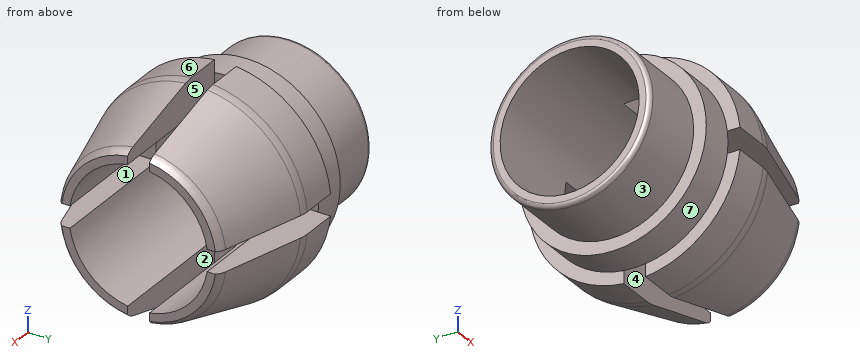
from build123d import *

# Parameters (mm, degrees)
F2_W          = 2.032
F2_H          = 3.556
F2_W_2        = 3.556
F2_H_2        = 2.032
F3_DEPTH      = 25.4
F3_DEPTH_BACK = 4.3434


# Not quite as in the source:
# - a feature names something its author has since deleted; it is built from what else it names


with BuildPart() as f1:
    # F0 (on Front) → F1 (revolve)
    with BuildSketch(Plane.XZ):
        with BuildLine():
            ThreePointArc((8.3732076521, 7.2620277332), (8.0243377529, 7.5505761386), (7.608205325, 7.728913435))
            Line((7.608205325, 7.728913435), (-0.1130385595, 9.7978144985))
            ThreePointArc((-0.1130385595, 9.7978144985), (-0.5203683675, 9.8788374349), (-0.9347890277, 9.906))
            Line((-0.9347890277, 9.906), (-4.3267923479, 9.906))
            Line((-4.3267923479, 9.906), (-4.3267923479, 8.73125))
            Line((-4.3267923479, 8.73125), (-7.5017923479, 8.73125))
            Line((-7.5017923479, 8.73125), (-7.5017923479, 7.5438))
            Line((-7.5017923479, 7.5438), (-13.4549173479, 7.5438))
            ThreePointArc((-13.4549173479, 7.5438), (-13.7355503517, 7.4275580038), (-13.8517923479, 7.146925))
            Line((-13.8517923479, 7.146925), (-13.8517923479, 6.5024))
            Line((-13.8517923479, 6.5024), (8.3732076521, 6.5024))
            Line((8.3732076521, 6.5024), (8.3732076521, 7.2620277332))
        make_face()
    revolve(axis=Axis((-0.2325048039, 0, 0), (1, 0, 0)))

    # F2 (on Right) → F3 (cut, two sides)
    with BuildSketch(Plane.YZ) as f3_sk:
        with Locations((0, -8.1534)):
            Rectangle(F2_W, F2_H)
        with Locations((0, 8.1534)):
            Rectangle(F2_W, F2_H)
        with Locations((-8.1534, 0)):
            Rectangle(F2_W_2, F2_H_2)
        with Locations((8.1534, 0)):
            Rectangle(F2_W_2, F2_H_2)
    extrude(amount=F3_DEPTH, mode=Mode.SUBTRACT)
    extrude(f3_sk.sketch, amount=-F3_DEPTH_BACK, mode=Mode.SUBTRACT)


solid = f1.part
The listing builds one solid part. Answer for the finished solid, in the listing's coordinates (mm). Face numbers are marked on the shaded views. A direction names the side the tool comes from. Round coordinates to 2 decimals unless told otherwise and drop trailing zeros. Write each loop counter-clockwise with the first axis right and the second up, starting at its lowest first coordinate (ties: lowest second). Pieces come first, ordered by that corner, then holes. Notation, with made-up numbers: M 76.5,38.25 L 125.5,38.25 A15 cw 125.5,53.25 Z; hole C 81.5,14.5 d6. An arc over 180 degrees is marked long. Write each question's results on one line, items separated by ' | '. Start each with the question number.
Item 1: The mould has two halves that part along Y. Classify the marked faces 4, 5, 6 and 7: +Y half, -Y half, draft (parallel to the pull), parting line (faces both ways), or undercut.
Item 2: Find section D-D on x = -7. Write down the section's boundary in (y, z), and give its area (3 significant figures).
Item 3: Find section A-A on z = 0. Write down the section's boundary in (x, y).
Item 4: Find section B-B on x = 7. Write down the section's boundary in (y, z), and give its area (3 significant figures).
Item 5: Straight lines are drawn through the part: probe 1 along Z at (x, y) = (-7.25, 0); probe 2 along X at (y, z) = (0.5, 7); probe 3 along Y at (x, z) = (3, 1.25). For each, find the intervals that lie inside material, in ascending order.
Item 6: Given pin 1 Ø10 at (x, z) = (1, 7.5) entering from +Y; pin 2 Ø2.5 at (x, z) = (0.5, 8) entering from -Y; pin 3 Ø4 at (x, y) = (2.5, 8.5) entering from -Z, each flat-ended and moving along its own axis, determine where each tip first touches the part or whether it passes through.
Item 7: Which of the six approach directions +Z, -Z, +X, -X, +Y, -Y give full straight-line access (tool end or side, diameter ignored) to the marked faces 1, 2 and 3?
Answer block:
1) face 4: undercut | face 5: undercut | face 6: -Y half | face 7: parting line
2) outline: C 0,0 d17.46; hole C 0,0 d13 | area: 107 mm²
3) outline: M -13.85,-7.15 A0.4 ccw -13.45,-7.54 L -7.5,-7.54 L -7.5,-8.73 L -4.34,-8.73 L -4.34,-6.5 L -13.85,-6.5 Z; M -13.85,6.5 L -4.34,6.5 L -4.34,8.73 L -7.5,8.73 L -7.5,7.54 L -13.45,7.54 A0.4 ccw -13.85,7.15 Z
4) outline: M -7.83,-1.02 A7.89 ccw -1.02,-7.83 L -1.02,-6.42 A6.5 cw -6.42,-1.02 Z; M -7.83,1.02 L -6.42,1.02 A6.5 cw -1.02,6.42 L -1.02,7.83 A7.89 ccw Z; M 1.02,-7.83 A7.89 ccw 7.83,-1.02 L 6.42,-1.02 A6.5 cw 1.02,-6.42 Z; M 1.02,6.42 A6.5 cw 6.42,1.02 L 7.83,1.02 A7.89 ccw 1.02,7.83 Z | area: 51.5 mm²
5) probe 1: z = -8.73 to -6.5, 6.5 to 8.73 | probe 2: x = -13.85 to -4.34 | probe 3: y = -8.88 to -6.38, 6.38 to 8.88
6) pin 1: stops at y = 9.49 | pin 2: stops at y = -6.96 | pin 3: stops at z = -6.5
7) face 1: +X, +Y, -Y | face 2: +Z, -Z, +X | face 3: -X
